```python
from build123d import *

# Parameters (mm, degrees)
SKETCH1_W                 = 430
SKETCH1_H                 = 60
BOSS_EXTRUDE1_DEPTH       = 3
OTW_R_POD_RUB_M31_D       = 3.4
SKETCH4_R                 = 7.5
CUT_EXTRUDE1_DEPTH        = 5
F_3_0MM_DOWEL_HOLE1_D     = 3
F_3_0MM_DOWEL_HOLE1_DEPTH = 6
F_3_0MM_DOWEL_HOLE1_TIP   = 0.901290929


with BuildPart() as part:
    # Sketch1 → Boss-Extrude1 (new body)
    with BuildSketch(Plane(origin=(0, 0, 0), x_dir=(1, 0, 0), z_dir=(0, 1, 0))):
        with Locations((85, 30)):
            Rectangle(SKETCH1_W, SKETCH1_H)
    extrude(amount=BOSS_EXTRUDE1_DEPTH)

    # Otwór pod śrubę M31 (through all)
    with Locations(Plane(origin=(0, 3, 0), x_dir=(1, 0, 0), z_dir=(0, 1, 0))):
        with Locations((266, 34), (24, 34), (125, 15), (165, 15), (165, 45), (125, 45)):
            Hole(OTW_R_POD_RUB_M31_D / 2)

    # Sketch4 → Cut-Extrude1 (cut)
    with BuildSketch(Plane(origin=(0, 3, 0), x_dir=(1, 0, 0), z_dir=(0, 1, 0))):
        with Locations(Location((-113, 30, 0), (0, 0, 270))):
            Circle(SKETCH4_R)
    extrude(amount=-CUT_EXTRUDE1_DEPTH, mode=Mode.SUBTRACT)

    # Ø3.0mm Dowel Hole1
    with Locations(Plane(origin=(0, 3, 0), x_dir=(1, 0, 0), z_dir=(0, 1, 0))):
        with Locations((-104.514718626, 21.514718626), (-104.514718626, 38.485281374), (-121.485281374, 21.514718626), (-121.485281374, 38.485281374)):
            Hole(F_3_0MM_DOWEL_HOLE1_D / 2, depth=F_3_0MM_DOWEL_HOLE1_DEPTH)
            with Locations((0, 0, -(F_3_0MM_DOWEL_HOLE1_DEPTH + F_3_0MM_DOWEL_HOLE1_TIP / 2))):  # 118° drill point
                Cone(0, F_3_0MM_DOWEL_HOLE1_D / 2, F_3_0MM_DOWEL_HOLE1_TIP, mode=Mode.SUBTRACT)


solid = part.part
```
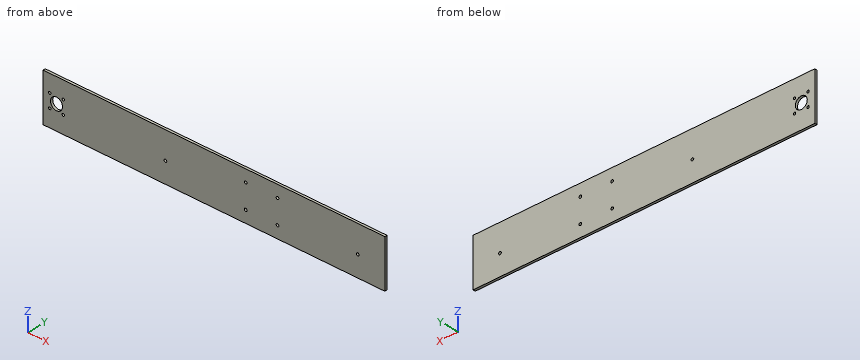
For this review, take the finished solid that the model builds, in its own axes (mm). Round coordinates to 2 decimals unless told otherwise and drop trailing zeros. Write each loop counter-clockwise with the first axis right and the second up, starting at its lowest first coordinate (ties: lowest second). Pieces come first, ordered by that corner, then holes.
1) Insertion check: pin 1 Ø5 at (x, z) = (-121.49, -21.51) entering from -Y. The pin has a flat end and moves straight along its axis. Give the tip position at first contact, or say it passes through.
Answer below:
pin 1: stops at y = 0
2) Take a section at A-A on x = -113. Give the boundary of the cut face in (y, z).
Answer below:
outline: (0, -60) - (3, -60) - (3, -37.5) - (0, -37.5) - close; (0, -22.5) - (3, -22.5) - (3, 0) - (0, 0) - close
3) For line 1 along Z through (x, y) = (165, 1.15); line 2 along X through (y, z) = (0.2, -44); line 3 along X through (y, z) = (1.1, -33), list the stretches that pass through material, from the lowest coordinate up.
Answer below:
line 1: z = -60 to -46.7, -43.3 to -16.7, -13.3 to 0
line 2: x = -130 to 123.63, 126.37 to 163.63, 166.37 to 300
line 3: x = -130 to -119.87, -106.13 to 22.63, 25.37 to 264.63, 267.37 to 300
